from build123d import *

# Parameters (mm, degrees)
SKETCH1_R      = 2.35
SKETCH1_R_2    = 1
EXTRUDE1_DEPTH = 2


with BuildPart() as part:
    # Sketch1 → Extrude1 (new body)
    with BuildSketch(Plane(origin=(0, 0, 0), x_dir=(1, 0, 0), z_dir=(0, 1, 0))):
        with BuildLine():
            Line((-5.186041147, 3.316192399), (2.637731834, -10.234979911))
            ThreePointArc((2.637731834, -10.234979911), (4.802795343, -11.484979911), (6.967858853, -10.234979911))
            Line((6.967858853, -10.234979911), (14.791631834, 3.316192399))
            ThreePointArc((14.791631834, 3.316192399), (14.791631834, 5.816192399), (12.626568324, 7.066192399))
            Line((12.626568324, 7.066192399), (-3.020977638, 7.066192399))
            ThreePointArc((-3.020977638, 7.066192399), (-5.186041147, 5.816192399), (-5.186041147, 3.316192399))
        make_face()
        with Locations((-2.110635714, 4.040606244)):
            Circle(SKETCH1_R, mode=Mode.SUBTRACT)
        with Locations((4.802795343, -7.933807601)):
            Circle(SKETCH1_R, mode=Mode.SUBTRACT)
        with Locations((11.7162264, 4.040606244)):
            Circle(SKETCH1_R, mode=Mode.SUBTRACT)
        with Locations((1.270334632, 2.088602105)):
            Circle(SKETCH1_R_2, mode=Mode.SUBTRACT)
        with Locations((4.770334632, 2.088602105)):
            Circle(SKETCH1_R_2, mode=Mode.SUBTRACT)
        with Locations((8.270334632, 2.088602105)):
            Circle(SKETCH1_R_2, mode=Mode.SUBTRACT)
        with Locations((1.270334632, -1.411397895)):
            Circle(SKETCH1_R_2, mode=Mode.SUBTRACT)
        with Locations((4.770334632, -1.411397895)):
            Circle(SKETCH1_R_2, mode=Mode.SUBTRACT)
        with Locations((8.270334632, -1.411397895)):
            Circle(SKETCH1_R_2, mode=Mode.SUBTRACT)
        with Locations((1.270334632, -4.911397895)):
            Circle(SKETCH1_R_2, mode=Mode.SUBTRACT)
        with Locations((8.270334632, -4.911397895)):
            Circle(SKETCH1_R_2, mode=Mode.SUBTRACT)
    extrude(amount=EXTRUDE1_DEPTH)


solid = part.part
The listing builds one solid part. Answer for the finished solid, in the listing's coordinates (mm). Give positions to 0.01 mm unless a question says otherwise; leave off trailing zeros. Loops run counter-clockwise (first coordinate to the right, second up) from the corner with the lowest first, then second, coordinate; pieces in that order, holes last.
Item 1: A cutting plane is placed at D-D (y = 0.35). Give the number of separate pieces and of enclosed holes in the cut face, then the cut area to 3 significant figures.
Derived:
separate pieces: 1
enclosed holes: 11
area: 166 mm2
Item 2: A cutting plane is placed at C-C (x = 7.5). Give the vertices of the cut face in (y, z).
Derived:
outline: (0, -7.07) - (2, -7.07) - (2, -2.73) - (0, -2.73) - close; (0, -1.45) - (2, -1.45) - (2, 0.77) - (0, 0.77) - close; (0, 2.05) - (2, 2.05) - (2, 4.27) - (0, 4.27) - close; (0, 5.55) - (2, 5.55) - (2, 9.31) - (0, 9.31) - close
Item 3: Each of these flat-tipped pins is pushed along its axis until it touches: pin 1 Ø1.2 at (x, z) = (8.27, 4.91) entering from -Y; pin 2 Ø3 at (x, z) = (1.27, 1.41) entering from -Y. Where does it stop, or does it pass through?
Derived:
pin 1: passes through
pin 2: stops at y = 0
Item 4: Find the intervals of material crossed by line 1 along X through (y, z) = (1.85, -5.75); line 2 along X through (y, z) = (1.5, 4.5); line 3 along Z through (x, y) = (0.5, 1.4), in increasing order.
Derived:
line 1: x = -5.22 to -3.72, -0.5 to 10.1, 13.33 to 14.83
line 2: x = -0.67 to 0.36, 2.18 to 7.36, 9.18 to 10.28
line 3: z = -7.07 to -2.73, -1.45 to 0.77, 2.05 to 4.27, 5.55 to 6.53
Item 5: A cutting plane is placed at B-B (z = 7.25). Give the vertices of the cut face in (x, y).
Derived:
outline: (0.91, 0) - (2.55, 0) - (2.55, 2) - (0.91, 2) - close; (7.05, 0) - (8.69, 0) - (8.69, 2) - (7.05, 2) - close
Item 6: Determine the mould class of faces 1 (the cylindrical face through (14.8, 1, -5.8)), 2 (the cylindrical face through (4.497, 0.986, 5.604)), 3 (the cylindrical face through (-5.167, 0.986, -5.848)) for opening direction X: +X half, -X half, draft (parallel to the pull), parting line (faces both ways), or undercut.
Derived:
face 1: +X half
face 2: undercut
face 3: -X half
Item 7: A cutting plane is placed at A-A (x = -3.75). Give the vertices of the cut face in (y, z), then the cut area to 3 significant figures.
Derived:
outline: (0, -6.96) - (2, -6.96) - (2, -5.72) - (0, -5.72) - close; (0, -2.36) - (2, -2.36) - (2, -0.83) - (0, -0.83) - close
area: 5.52 mm2
